Input: dimensioned drawing with shaded views. Units: mm. Origin: part minimum x, y, z. Round coordinates to 2 decimals unless told otherwise and drop trailing zeros. Loops run counter-clockwise (first coordinate to the right, second up) from the corner with the lowest first, then second, coordinate; pieces in that order, holes last. Notation, with made-up numbers: M 30,60.5 L 56,60.5 A7 cw 56,66.5 Z; hole C -17,56 d2. An arc over 180 degrees is marked long. Return JSON: item names as keys, results as strings.
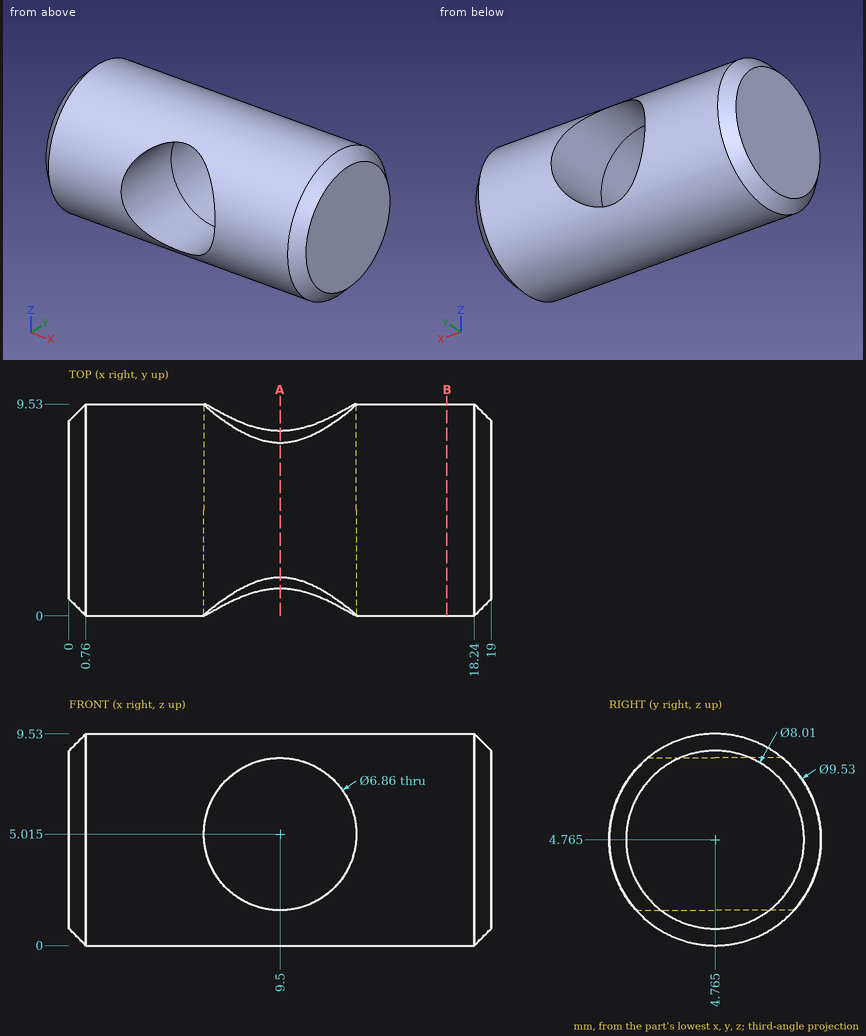
Q1. Section query A-A (x = 9.5). Output: boundary loops of the cut face in (y, z) (3 decimals), plus the area to 3 significant figures.
Determined:
{"outline": "M 1.216,1.585 A4.765 ccw 8.314,1.585 Z; M 1.738,8.445 L 7.792,8.445 A4.765 ccw Z", "area": "12.3 mm^2"}
Q2. Pin query (flat end, axial travel): pin 1 (1 mm diameter, centred on y = 2, z = 1, fed in from -X); pin 2 (5 mm diameter, centred on x = 5.5, y = 7.5, fed in from +Z). Return the tip coordinate at first contact, or that it passes through.
Determined:
{"pin 1": "stops at x = 0.17", "pin 2": "stops at z = 9.52"}
Q3. Section query B-B (x = 17). Output: boundary loops of the cut face in (y, z) (3 decimals).
Determined:
{"outline": "C 4.765,4.765 d9.53"}
Q4. Material intervals for L1, parallel to Z at x = 9.5, y = 7.4 (3 decimals); L2, parallel to Z at x = 9.5, y = 3.2 (3 decimals); L3, parallel to X at y = 2.25, z = 5.25, sorted ascending.
Determined:
{"L1": "z = 0.795 to 1.585, 8.445 to 8.735", "L2": "z = 0.264 to 1.585, 8.445 to 9.266", "L3": "x = 0 to 6.08, 12.92 to 19"}
